Check sheet for the modelled part. Datum: model origin and axes. Units: mm. A direction names the side the tool comes from. Coordinates: 2 decimals unless noted, no trailing zeros. Write each loop counter-clockwise with the first axis right and the second up, starting at its lowest first coordinate (ties: lowest second). Pieces come first, ordered by that corner, then holes. Notation, with made-up numbers: (42, 9) - (70, 9) arc R13 cw to (70, 19) - close; hole circle Ø8 at (82.25, -4.75). An arc over 180 degrees is marked (long way). Use one line per item in the form item = value. Start each with the question number.
1. Scan lines: line 1 along X through (y, z) = (15, 16) (3 decimals); line 2 along Z through (x, y) = (-26.5, 7); line 3 along Y through (x, z) = (-30, 7.5). Record each from-to range of solid material in increasing order.
2. Go/stop test with flat-tipped pins: pin 1 Ø4 at (x, z) = (-1, 30) entering from -Y; pin 2 Ø5 at (x, y) = (-10.5, 4) entering from +Z; pin 3 Ø8 at (x, y) = (12.5, -36.5) entering from -Z; pin 4 Ø2 at (y, z) = (-24.5, 8.5) entering from -X (3 decimals). Record where each tip stops, or that it passes through.
3. Draft check along Y on faces 1 (the face through (0, 19.05, 20)), 2 (the face through (38.01, -36.6, 18.63)), 3 (the face through (-1, 21.59, 19)). Enter one of: +Y half, -Y half, draft (parallel to the pull), parting line (faces both ways), or undercut.
4. Cross-section at B-B on x = -20. Record the boundary of the cut face in (y, z), then the cut area to 3 significant figures.
5. Cross-section at A-A on y = 8.5. Record the boundary of the cut face in (x, z) (3 decimals).
6. Tool access check on faces 4 (the face through (0.51, -37.63, 18.58)), 5 (the face through (0, 0, 5.08)). Record the directions out of +Z, -Z, +X, -X, +Y, -Y that give a thin tool (end or side, any length) a straight path to the whole face; none if there is none.
```python
from build123d import *

# Parameters (mm, degrees)
SKETCH1_W           = 69.85
SKETCH1_H           = 38.1
BOSS_EXTRUDE1_DEPTH = 5.08
BOSS_EXTRUDE2_DEPTH = 69.85
BOSS_EXTRUDE3_DEPTH = 3.81
BOSS_EXTRUDE4_DEPTH = 3.81
SKETCH6_W           = 77.47
SKETCH6_H           = 35.921024484
BOSS_EXTRUDE5_DEPTH = 2.54
FILLET1_R           = 2.54
CUT_EXTRUDE1_DEPTH  = 2.54


with BuildPart() as part:
    # Sketch1 → Boss-Extrude1 (new body)
    with BuildSketch(Plane.XY):
        Rectangle(SKETCH1_W, SKETCH1_H)
    extrude(amount=BOSS_EXTRUDE1_DEPTH)

    # Sketch2 → Boss-Extrude2 (add)
    with BuildSketch(Plane.ZY.offset(34.925)):
        Polygon((5.08, -19.05), (20.200368371, -34.170368371), (29.556522172, -43.526522172), (35.921024484, -49.891024484), (35.921024484, -54.971024484), (0, -19.05), align=None)
    extrude(amount=-BOSS_EXTRUDE2_DEPTH)

    # Sketch3 → Boss-Extrude3 (add)
    with BuildSketch(Plane(origin=(34.925, 0, 0), x_dir=(0, 0, -1), z_dir=(1, 0, 0))):
        Polygon((-35.921024484, -54.971024484), (0, -19.05), (0, 19.05), (-35.921024484, 19.05), align=None)
    extrude(amount=BOSS_EXTRUDE3_DEPTH)

    # Sketch5 → Boss-Extrude4 (add)
    with BuildSketch(Plane.ZY.offset(34.925)):
        Polygon((5.08, 19.05), (35.921024484, 19.05), (35.921024484, -54.971024484), (0, -19.05), (0, 19.05), align=None)
    extrude(amount=BOSS_EXTRUDE4_DEPTH)

    # Sketch6 → Boss-Extrude5 (add)
    with BuildSketch(Plane(origin=(0, 19.05, 0), x_dir=(1, 0, 0), z_dir=(0, 1, 0))):
        with Locations((0, -17.960512242)):
            Rectangle(SKETCH6_W, SKETCH6_H)
    extrude(amount=BOSS_EXTRUDE5_DEPTH)

    # Fillet1
    fillet1_edges = [part.edges().sort_by_distance(p)[0] for p in [
        (38.735, -37.010512242, 17.960512242),
        (38.735, 1.27, 0),
        (-38.735, 1.27, 0),
        (-38.735, -37.010512242, 17.960512242),
        (0, -19.05, 0),
        (38.735, 21.59, 17.960512242),
        (0, 21.59, 0),
        (-38.735, 21.59, 17.960512242),
    ]]
    fillet(fillet1_edges, radius=FILLET1_R)

    # Sketch7 → Cut-Extrude1 (cut)
    with BuildSketch(Plane(origin=(0, 21.59, 0), x_dir=(1, 0, 0), z_dir=(0, 1, 0))):
        with BuildLine():
            ThreePointArc((5.483864, -12.7), (4.898077562, -11.285786438), (3.483864, -10.7))
            Line((3.483864, -10.7), (3.483864, -14.7))
            ThreePointArc((3.483864, -14.7), (4.898077562, -14.114213562), (5.483864, -12.7))
        make_face()
        with BuildLine():
            Line((3.483864, -14.7), (3.483864, -10.7))
            ThreePointArc((3.483864, -10.7), (1.483864, -12.7), (3.483864, -14.7))
        make_face()
        with BuildLine():
            ThreePointArc((5.483864, -30.079024484), (4.898077562, -28.664810922), (3.483864, -28.079024484))
            Line((3.483864, -28.079024484), (3.483864, -32.079024484))
            ThreePointArc((3.483864, -32.079024484), (4.898077562, -31.493238047), (5.483864, -30.079024484))
        make_face()
        with BuildLine():
            Line((3.483864, -32.079024484), (3.483864, -28.079024484))
            ThreePointArc((3.483864, -28.079024484), (1.483864, -30.079024484), (3.483864, -32.079024484))
        make_face()
    extrude(amount=-CUT_EXTRUDE1_DEPTH, mode=Mode.SUBTRACT)


solid = part.part
```
Final values:
q1.line_1 = -38.735 to -34.925, 34.925 to 38.735
q1.line_2 = 0 to 5.08
q1.line_3 = -26.55 to -21.47, 19.05 to 21.59
q2.pin_1 = -51.05
q2.pin_2 = 5.08
q2.pin_3 = 13.45
q2.pin_4 = -38.735
q3.face_1 = undercut
q3.face_2 = -Y half
q3.face_3 = +Y half
q4.outline = (-54.97, 35.92) - (-19.79, 0.74) arc R2.54 ccw to (-18, 0) - (19.05, 0) arc R2.54 ccw to (21.59, 2.54) - (21.59, 35.92) - (19.05, 35.92) - (19.05, 5.08) - (-19.05, 5.08) - (-49.89, 35.92) - close
q4.area = 453 mm²
q5.outline = (-38.735, 2.54) arc R2.54 ccw to (-36.195, 0) - (36.195, 0) arc R2.54 ccw to (38.735, 2.54) - (38.735, 35.921) - (34.925, 35.921) - (34.925, 5.08) - (-34.925, 5.08) - (-34.925, 35.921) - (-38.735, 35.921) - close
q6.face_4 = -Z, +X, -X, -Y
q6.face_5 = +Z
